Read the model definition and answer for the solid it produces. Units are mm, in the model's axes. A direction names the side the tool comes from. Give positions to 0.01 mm unless a question says otherwise; leave off trailing zeros. Loops run counter-clockwise (first coordinate to the right, second up) from the corner with the lowest first, then second, coordinate; pieces in that order, holes last. Notation, with made-up numbers: (-12, 70) - (28, 70) arc R11 cw to (28, 89) - close; hole circle Ø10 at (74.5, 31). An arc over 180 degrees is marked (long way). Use a Markdown table: item, result. Add a question column.
Item 1: Which of the six approach directions +Z, -Z, +X, -X, +Y, -Y give full straight-line access (tool end or side, diameter ignored) to faces 4 (the face through (20, 10, 1)), 5 (the face through (81, 10, 0)), 6 (the face through (5, 36, 40)), 7 (the face through (0, 40, -30))?
Item 2: For a pull along Z with two mould halves and no side action, classify faces 1 (the face through (5, 36, -40)), 2 (the face through (-10, 40, 0)), 3 (the face through (76, 52, 0)) as +Z half, -Z half, draft (parallel to the pull), parting line (faces both ways), or undercut.
Item 3: Each of these flat-tipped pins is pushed along its axis until it touches: P1, Ø1, axis at x = 86.5, y = 27, coming from the -Z side; P2, Ø5, axis at x = 65, y = 35, coming from the -Z side; P3, Ø6, axis at y = 9, z = 0, coming from the -X side. Where does it stop, or does it pass through?
Item 4: A cutting plane is placed at C-C (y = 24.5). Determine the outline of the cut face in (x, z), plus the area to 3 significant figures.
Item 5: A cutting plane is placed at A-A (x = 0). Determine the outline of the cut face in (y, z).
Item 6: A cutting plane is placed at D-D (z = -34). Determine the outline of the cut face in (x, y).
Item 7: Consider probe 1 along X at (y, z) = (36.5, -4); probe 2 along Y at (x, z) = (15.5, -34); probe 3 along X at (y, z) = (29, 11.5). Determine where each line is inside the solid, lowest interval first. Write a range as [from, to].
Item 8: A cutting plane is placed at B-B (z = 6.5). Determine the outline of the cut face in (x, y).
from build123d import *

# Parameters (mm, degrees)
SKETCH1_W           = 40
SKETCH1_H           = 80
SKETCH1_W_2         = 10
BOSS_EXTRUDE1_DEPTH = 60
SKETCH2_W           = 40
SKETCH2_H           = 20
CUT_EXTRUDE1_DEPTH  = 81
CUT_EXTRUDE2_DEPTH  = 10
CUT_EXTRUDE3_DEPTH  = 61
CUT_EXTRUDE4_DEPTH  = 81


with BuildPart() as part:
    # Sketch1 → Boss-Extrude1 (new body)
    with BuildSketch(Plane(origin=(0, 0, 0), x_dir=(1, 0, 0), z_dir=(0, 1, 0))):
        Rectangle(SKETCH1_W, SKETCH1_H)
        Polygon((100, -10), (30, -40), (30, 40), (100, 10), align=None)
        with Locations((25, 0)):
            Rectangle(SKETCH1_W_2, SKETCH1_H)
    extrude(amount=BOSS_EXTRUDE1_DEPTH)

    # Sketch2 → Cut-Extrude1 (cut, through all)
    with BuildSketch(Plane.XY.offset(40)):
        with Locations((0, 10)):
            Rectangle(SKETCH2_W, SKETCH2_H)
    extrude(amount=-CUT_EXTRUDE1_DEPTH, mode=Mode.SUBTRACT)

    # Sketch3 → Cut-Extrude2 (cut)
    with BuildSketch(Plane.XZ):
        Polygon((70, 0), (100, 0), (100, 10), (70, 22.857142857), align=None)
        Polygon((100, -10), (100, 0), (70, 0), (70, -22.857142857), align=None)
    extrude(amount=-CUT_EXTRUDE2_DEPTH, mode=Mode.SUBTRACT)

    # Sketch5 → Cut-Extrude3 (cut, through all)
    with BuildSketch(Plane(origin=(0, 60, 0), x_dir=(1, 0, 0), z_dir=(0, 1, 0))):
        with BuildLine():
            Line((-10, -20), (-10, 20))
            ThreePointArc((-10, 20), (0, 30), (10, 20))
            Line((10, 20), (10, -20))
            ThreePointArc((10, -20), (0, -30), (-10, -20))
        make_face()
    extrude(amount=-CUT_EXTRUDE3_DEPTH, mode=Mode.SUBTRACT)

    # Sketch6 → Cut-Extrude4 (cut, through all)
    with BuildSketch(Plane.XY.offset(40)):
        Polygon((60, 60), (100, 60), (100, 40), align=None)
    extrude(amount=-CUT_EXTRUDE4_DEPTH, mode=Mode.SUBTRACT)


solid = part.part
Geometry says:
| question | item | result |
|---|---|---|
| 1 | face 4 | +Z, -Z, -X, -Y |
| 1 | face 5 | +Z, -Z, +X, -Y |
| 1 | face 6 | +Z, +X, -X, +Y, -Y |
| 1 | face 7 | +Y, -Y |
| 2 | face 1 | -Z half |
| 2 | face 2 | undercut |
| 2 | face 3 | draft |
| 3 | P1 | z = -16 |
| 3 | P2 | z = -26.07 |
| 3 | P3 | x = 20 |
| 4 | outline | (-20, -40) - (30, -40) - (100, -10) - (100, 10) - (30, 40) - (-20, 40) - close; hole (-10, -20) arc R10 ccw to (10, -20) - (10, 20) arc R10 ccw to (-10, 20) - close |
| 4 | area | 6,390 mm² |
| 5 | outline | (20, -40) - (60, -40) - (60, -30) - (20, -30) - close; (20, 30) - (60, 30) - (60, 40) - (20, 40) - close |
| 6 | outline | (-20, 20) - (20, 20) - (20, 0) - (44, 0) - (44, 60) - (-20, 60) - close |
| 7 | probe 1 | [-20, -10], [10, 100] |
| 7 | probe 2 | [20, 60] |
| 7 | probe 3 | [-20, -10], [10, 96.5] |
| 8 | outline | (-20, 20) - (-10, 20) - (-10, 60) - (-20, 60) - close; (10, 20) - (20, 20) - (20, 0) - (70, 0) - (70, 10) - (100, 10) - (100, 40) - (60, 60) - (10, 60) - close |
